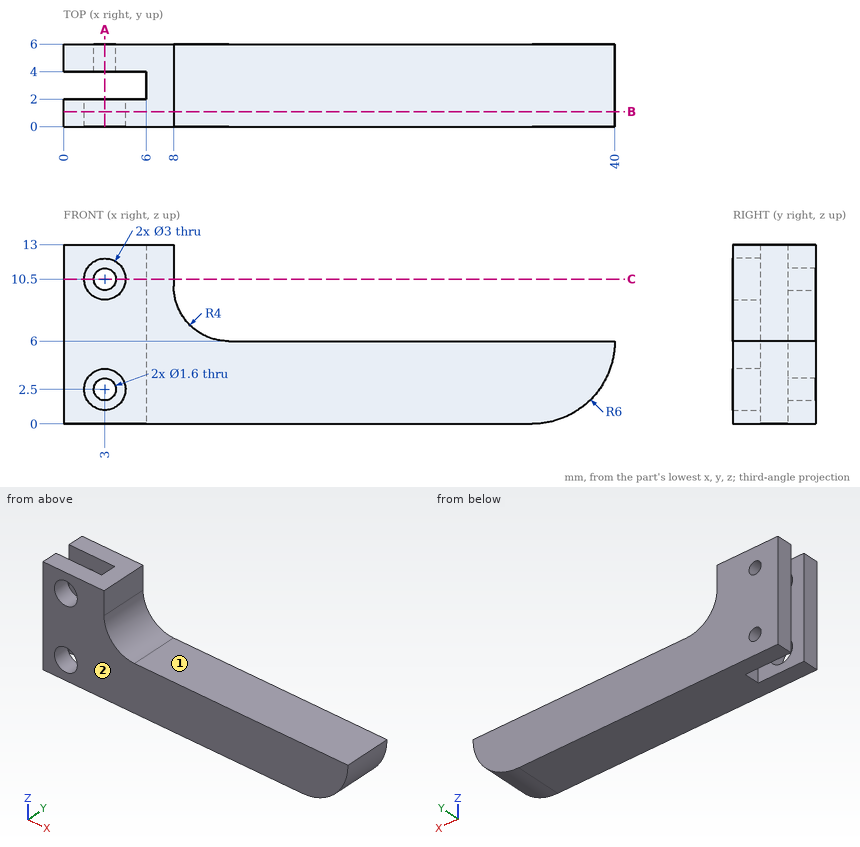
Could you check a few things on this drawing? It's one solid part, dimensions in mm from its lowest x, y, z. A direction names the side the tool comes from. Round coordinates to 2 decimals unless told otherwise and drop trailing zeros. Loops run counter-clockwise (first coordinate to the right, second up) from the corner with the lowest first, then second, coordinate; pieces in that order, holes last. Notation, with made-up numbers: M 44.5,66.25 L 60.5,66.25 A15 ccw 60.5,89.25 Z; hole C 53.5,30 d5. An arc over 180 degrees is marked long. Write item = value, one per line. Start each with the question number.
(1) Which directions (+Z, -Z, +X, -X, +Y, -Y) give clear straight access to the entire face, cutting with the end or side of a thin tool? Please do the marked faces 1 and 2.
(2) I need wall thicknesses on line 1 along Y through (x, z) = (5, 11.5); line 2 along X through (y, z) = (0.4, 10.5); line 3 along Z through (x, y) = (23, 0.75). Which ranges of each line are inside material? Lowest first, please.
(3) Suppose I cut it at A-A on x = 3. Write out the boundary of the cut face in (y, z).
(4) Suppose I cut it at B-B on y = 1.1. Give the number of separate pieces and of enclosed holes in the cut face, plus the area to 3 significant figures.
(5) I'm going to push flat-ended pins straight in: P1, Ø2, axis at x = 21.5, y = 1.5, coming from the +Z side; P2, Ø0.9, axis at y = 3, z = 11, coming from the +X side; P3, Ø2.5, axis at x = 3, z = 10.5, coming from the -Y side. Where does each tip first touch, or does it pass through?
(6) Suppose I cut it at C-C on z = 10.5. Write out the boundary of the cut face in (x, y), plus the area to 3 significant figures.
Answer block:
q1.face_1 = +Z, +X, +Y, -Y
q1.face_2 = +Z, -Z, +X, -X, -Y
q2.line_1 = 0 to 2, 4 to 6
q2.line_2 = 0 to 1.5, 4.5 to 8
q2.line_3 = 0 to 6
q3.outline = M 0,0 L 2,0 L 2,1 L 0,1 Z; M 0,4 L 2,4 L 2,9 L 0,9 Z; M 0,12 L 2,12 L 2,13 L 0,13 Z; M 4,0 L 6,0 L 6,1.7 L 4,1.7 Z; M 4,3.3 L 6,3.3 L 6,9.7 L 4,9.7 Z; M 4,11.3 L 6,11.3 L 6,13 L 4,13 Z
q4.separate_pieces = 1
q4.enclosed_holes = 2
q4.area = 278 mm²
q5.P1 = 6
q5.P2 = 8
q5.P3 = 4
q6.outline = M 0,0 L 1.5,0 L 1.5,2 L 0,2 Z; M 0,4 L 2.2,4 L 2.2,6 L 0,6 Z; M 3.8,4 L 6,4 L 6,2 L 4.5,2 L 4.5,0 L 8,0 L 8,6 L 3.8,6 Z
q6.area = 26.8 mm²
